Source: CAD feature listing. Evaluate the final solid. Frame: model axes, mm. A direction names the side the tool comes from. Give positions to 0.01 mm unless a question says otherwise; leave off trailing zeros. Order: outer loops, then holes, each group sorted by start corner. A loop starts at its lowest first (then second) coordinate and runs counter-clockwise, first axis right, second up. Notation, with made-up numbers: (-8.5, 75) - (20.5, 75) arc R10 ccw to (20.5, 88) - close; hole circle Ø7 at (-26, -1). An arc over 180 degrees is marked (long way). Use CSV: the item, a comma, the result in double quotes.
```python
from build123d import *

# Parameters (mm, degrees)
SKETCH1_R           = 1
BOSS_EXTRUDE3_DEPTH = 2


with BuildPart() as part:
    # Sketch1 → Boss-Extrude3 (new body)
    with BuildSketch(Plane.XY):
        Polygon((0, 4.973839636), (-0.426100438, 4.054074865), (-1.034119408, 4.865149306), (-1.259678681, 3.87689234), (-2.023042837, 4.543828606), (-2.038202921, 3.530271016), (-2.923549585, 4.023920792), (-2.727647913, 3.029359908), (-3.696283188, 3.328148331), (-3.297881603, 2.396051237), (-4.307471479, 2.486919818), (-3.723982041, 1.658023628), (-4.730402596, 1.537000975), (-3.987326594, 0.847532431), (-4.946592422, 0.519907814), (-4.076405843, 0), (-4.946592422, -0.519907814), (-3.987326594, -0.847532431), (-4.730402596, -1.537000975), (-3.723982041, -1.658023628), (-4.307471479, -2.486919818), (-3.297881603, -2.396051237), (-3.696283188, -3.328148331), (-2.727647913, -3.029359908), (-2.923549585, -4.023920792), (-2.038202921, -3.530271016), (-2.023042837, -4.543828606), (-1.259678681, -3.87689234), (-1.034119408, -4.865149306), (-0.426100438, -4.054074865), (0, -4.973839636), (0.426100438, -4.054074865), (1.034119408, -4.865149306), (1.259678681, -3.87689234), (2.023042837, -4.543828606), (2.038202921, -3.530271016), (2.923549585, -4.023920792), (2.727647913, -3.029359908), (3.696283188, -3.328148331), (3.297881603, -2.396051237), (4.307471479, -2.486919818), (3.723982041, -1.658023628), (4.730402596, -1.537000975), (3.987326594, -0.847532431), (4.946592422, -0.519907814), (4.076405843, 0), (4.946592422, 0.519907814), (3.987326594, 0.847532431), (4.730402596, 1.537000975), (3.723982041, 1.658023628), (4.307471479, 2.486919818), (3.297881603, 2.396051237), (3.696283188, 3.328148331), (2.727647913, 3.029359908), (2.923549585, 4.023920792), (2.038202921, 3.530271016), (2.023042837, 4.543828606), (1.259678681, 3.87689234), (1.034119408, 4.865149306), (0.426100438, 4.054074865), align=None)
        Circle(SKETCH1_R, mode=Mode.SUBTRACT)
    extrude(amount=BOSS_EXTRUDE3_DEPTH)


solid = part.part
```
Item 1: Mould query, pull axis X, two halves, no side actions, for faces 5 (the flat face through (3.22, 3.18, 0.99)), 6 (the flat face through (-4.02, 2.08, 0.99)), 7 (the flat face through (1.145, -4.378, 0.986)), 8 (the flat face through (4.51, 0.26, 0.99)). Classes: released by +X, released by -X, zero draft, split by the parting line, or undercut.
Filled in:
face 5,"undercut"
face 6,"released by -X"
face 7,"undercut"
face 8,"released by +X"
Item 2: Section C-C on y = -2.25. Return the cut outline in (x, z), then the cut area to 3 significant figures.
Filled in:
outline,"(-4.14, 0) - (4.14, 0) - (4.14, 2) - (-4.14, 2) - close"
area,"16.6 mm2"
Item 3: Material intervals for line 1 (X direction, y = 3.75, z = 1.85); line 2 (Y direction, x = -0.75, z = 0.85); line 3 (Y direction, x = 2.5, z = 1.3), sorted ascending. Write a range as from..to.
Filled in:
line 1,"x = -2.87..-2.43, -2.03..2.03, 2.43..2.87"
line 2,"y = -4.49..-0.66, 0.66..4.49"
line 3,"y = -3.79..3.79"
Item 4: Set-up query: faces 1 (the flat face through (-2.824, -3.52, 0.986)), 2 (the flat face through (2.47, -3.77, 0.99)), 3 (the flat face through (-4.474, -0.681, 0.986)), 4 (the flat face through (-1.145, 4.378, 0.986)). Return all of +Z, -Z, +X, -X, +Y, -Y with unobstructed straight access to the full face (end or side cutting, diameter ignored); none if empty.
Filled in:
face 1,"+Z, -Z"
face 2,"+Z, -Z, -Y"
face 3,"+Z, -Z, -X"
face 4,"+Z, -Z, +Y"
Item 5: Section A-A on y = 4.25. Return the cut outline in (x, z), then the cut area to 3 significant figures.
Filled in:
outline,"(-2.03, 0) - (-1.69, 0) - (-1.69, 2) - (-2.03, 2) - close; (-1.17, 0) - (-0.57, 0) - (-0.57, 2) - (-1.17, 2) - close; (-0.34, 0) - (0.34, 0) - (0.34, 2) - (-0.34, 2) - close; (0.57, 0) - (1.17, 0) - (1.17, 2) - (0.57, 2) - close; (1.69, 0) - (2.03, 0) - (2.03, 2) - (1.69, 2) - close"
area,"5.11 mm2"
Item 6: Section B-B on x = -3.5. Return the cut outline in (y, z).
Filled in:
outline,"(-3.27, 0) - (-2.87, 0) - (-2.87, 2) - (-3.27, 2) - close; (-2.41, 0) - (2.41, 0) - (2.41, 2) - (-2.41, 2) - close; (2.87, 0) - (3.27, 0) - (3.27, 2) - (2.87, 2) - close"
